```python
from build123d import *

# Parameters (mm, degrees)
BOSS_EXTRUDE1_DEPTH  = 5.6388
SKETCH2_W            = 63.5
SKETCH2_H            = 6.35
CUT_EXTRUDE1_DEPTH   = 6.6388
LPATTERN1_COUNT      = 4
LPATTERN1_PITCH      = 15.24
LPATTERN1_COUNT_DIR2 = 2
LPATTERN1_PITCH_DIR2 = 220
SKETCH3_W            = 25
SKETCH3_H            = 30
CUT_EXTRUDE2_DEPTH   = 6.6388
SKETCH4_W            = 38.1
SKETCH4_H            = 31.75
CUT_EXTRUDE3_DEPTH   = 6.6388


with BuildPart() as part:
    # Sketch1 → Boss-Extrude1 (new body)
    with BuildSketch(Plane(origin=(0, 0, 0), x_dir=(1, 0, 0), z_dir=(0, 1, 0))):
        Polygon((-185, -73.025), (185, -73.025), (185, -6.825), (185, 3.175), (175, 3.175), (-175, 3.175), (-185, 3.175), (-185, -6.825), align=None)
    extrude(amount=BOSS_EXTRUDE1_DEPTH)

    # Sketch2 → Cut-Extrude1 (cut, through all)
    with BuildSketch(Plane(origin=(0, 5.6388, 0), x_dir=(1, 0, 0), z_dir=(0, 1, 0))):
        with Locations((-83.25, -63.5)):
            Rectangle(SKETCH2_W, SKETCH2_H)
    cut_extrude1 = extrude(amount=-CUT_EXTRUDE1_DEPTH, mode=Mode.SUBTRACT)

    # LPattern1: Cut-Extrude1 4 × 2
    with Locations(*[(j * LPATTERN1_PITCH_DIR2, 0, -i * LPATTERN1_PITCH) for i in range(LPATTERN1_COUNT) for j in range(LPATTERN1_COUNT_DIR2) if (i, j) != (0, 0)]):
        add(cut_extrude1, mode=Mode.SUBTRACT)

    # Sketch3 → Cut-Extrude2 (cut, through all)
    with BuildSketch(Plane(origin=(0, 5.6388, 0), x_dir=(1, 0, 0), z_dir=(0, 1, 0))):
        with Locations((0, -58.025)):
            Rectangle(SKETCH3_W, SKETCH3_H)
    extrude(amount=-CUT_EXTRUDE2_DEPTH, mode=Mode.SUBTRACT)

    # Sketch4 → Cut-Extrude3 (cut, through all)
    with BuildSketch(Plane(origin=(0, 5.6388, 0), x_dir=(1, 0, 0), z_dir=(0, 1, 0))):
        with Locations((-143.95, -57.15)):
            Rectangle(SKETCH4_W, SKETCH4_H)
        with Locations((74.05, -57.15)):
            Rectangle(SKETCH4_W, SKETCH4_H)
    extrude(amount=-CUT_EXTRUDE3_DEPTH, mode=Mode.SUBTRACT)


solid = part.part
```
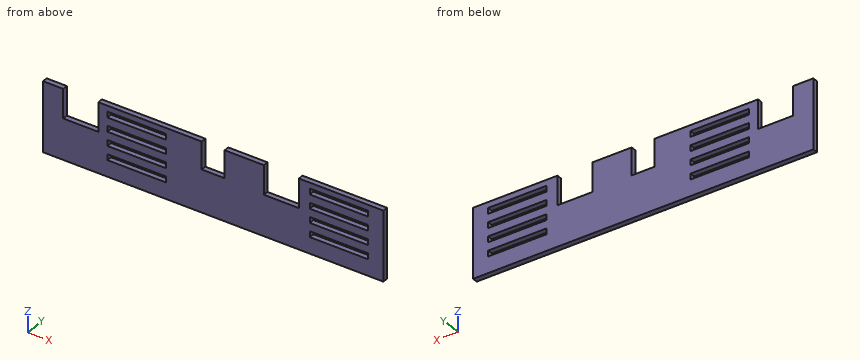
Geometry check sheet. Reference: the model listing, model coordinates, mm. Round coordinates to 2 decimals unless told otherwise and drop trailing zeros. Loops run counter-clockwise (first coordinate to the right, second up) from the corner with the lowest first, then second, coordinate; pieces in that order, holes last. Notation, with made-up numbers: (84.5, 8) -> (100.5, 8) arc R10 cw to (100.5, 26) -> close; hole circle Ø2 at (88.5, 27.5). An arc over 180 degrees is marked (long way). Use a Markdown table: item, result.
(1) Go/stop test with a flat-tipped pin: P1, Ø1.7, axis at x = -142.5, y = 1.5, coming from the +Z side (3 decimals). Record where the tip stops, or that it passes through.
Calculated:
| item | result |
|---|---|
| P1 | z = 41.275 |
(2) Scan lines: probe 1 along Z at (x, y) = (-101, 5.25) (3 decimals); probe 2 along X at (y, z) = (3.2, 34.5); probe 3 along X at (y, z) = (2.5, 45.5). Record each from-to range of solid material in increasing order.
Calculated:
| item | result |
|---|---|
| probe 1 | -3.175 to 14.605, 20.955 to 29.845, 36.195 to 45.085, 51.435 to 60.325, 66.675 to 73.025 |
| probe 2 | -185 to -115, -51.5 to 105, 168.5 to 185 |
| probe 3 | -185 to -163, -124.9 to -115, -51.5 to -12.5, 12.5 to 55, 93.1 to 105, 168.5 to 185 |
(3) Sectioned sample at C-C (y = 2.65). Give the number of separate pieces and of enclosed holes in the cut face, then the cut area to 3 significant figures.
Calculated:
| item | result |
|---|---|
| separate pieces | 1 |
| enclosed holes | 8 |
| area | 21,800 mm² |
(4) Sectioned sample at A-A (x = 127). Enter the section's corners in (y, z) (3 decimals).
Calculated:
| item | result |
|---|---|
| outline | (0, -3.175) -> (5.639, -3.175) -> (5.639, 14.605) -> (0, 14.605) -> close; (0, 20.955) -> (5.639, 20.955) -> (5.639, 29.845) -> (0, 29.845) -> close; (0, 36.195) -> (5.639, 36.195) -> (5.639, 45.085) -> (0, 45.085) -> close; (0, 51.435) -> (5.639, 51.435) -> (5.639, 60.325) -> (0, 60.325) -> close; (0, 66.675) -> (5.639, 66.675) -> (5.639, 73.025) -> (0, 73.025) -> close |
(5) Sectioned sample at D-D (x = -134.5). Enter the section's corners in (y, z) (3 decimals).
Calculated:
| item | result |
|---|---|
| outline | (0, -3.175) -> (5.639, -3.175) -> (5.639, 41.275) -> (0, 41.275) -> close |
(6) Sectioned sample at B-B (z = 57). Enter the section's corners in (x, y), then the cut area to 3 significant figures.
Calculated:
| item | result |
|---|---|
| outline | (-185, 0) -> (-163, 0) -> (-163, 5.64) -> (-185, 5.64) -> close; (-124.9, 0) -> (-12.5, 0) -> (-12.5, 5.64) -> (-124.9, 5.64) -> close; (12.5, 0) -> (55, 0) -> (55, 5.64) -> (12.5, 5.64) -> close; (93.1, 0) -> (185, 0) -> (185, 5.64) -> (93.1, 5.64) -> close |
| area | 1,520 mm² |
